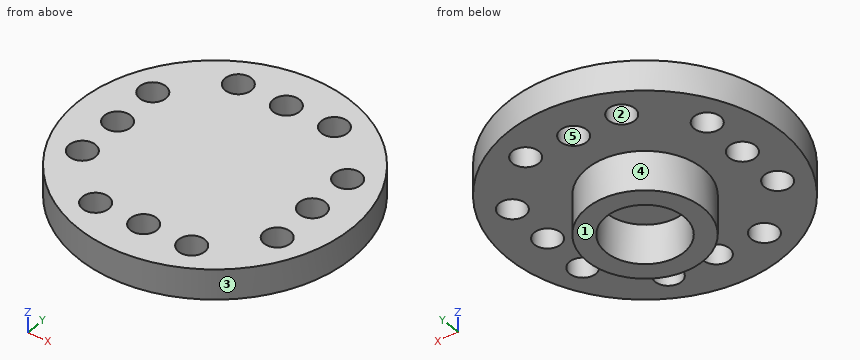
```python
from build123d import *

# Parameters (mm, degrees)
EXTRUDE_START       = 1
SKETCH_2_R          = 4.4
SKETCH_2_R_2        = 2.95
EXTRUDE_2_DEPTH     = 3
SKETCH_3_R          = 10.4
EXTRUDE_3_DEPTH     = 2.3
SKETCH_5_R          = 1
CUT_EXTRUDE_1_DEPTH = 2.3


with BuildPart() as part:
    # 스케치2 → 보스-돌출2 (new body)
    with BuildSketch(Plane.XY.offset(-4).offset(EXTRUDE_START)):
        with Locations((10.45, 0)):
            Circle(SKETCH_2_R)
        with Locations((10.45, 0)):
            Circle(SKETCH_2_R_2, mode=Mode.SUBTRACT)
    extrude(amount=EXTRUDE_2_DEPTH)

    # 스케치3 → 보스-돌출3 (add)
    with BuildSketch(Plane.XY):
        with Locations((10.45, 0)):
            Circle(SKETCH_3_R)
    extrude(amount=EXTRUDE_3_DEPTH)

    # 스케치5 → 컷-돌출1 (cut)
    with BuildSketch(Plane.XY.offset(2.3)):
        with Locations((10.45, 7.3)):
            Circle(SKETCH_5_R)
        with Locations((14.05, 7.3)):
            Circle(SKETCH_5_R)
        with Locations((6.85, 7.3)):
            Circle(SKETCH_5_R)
        with Locations((3.15, 0)):
            Circle(SKETCH_5_R)
        with Locations((3.15, 3.6)):
            Circle(SKETCH_5_R)
        with Locations((3.15, -3.6)):
            Circle(SKETCH_5_R)
        with Locations((10.45, -7.3)):
            Circle(SKETCH_5_R)
        with Locations((6.85, -7.3)):
            Circle(SKETCH_5_R)
        with Locations((14.05, -7.3)):
            Circle(SKETCH_5_R)
        with Locations((17.75, 0)):
            Circle(SKETCH_5_R)
        with Locations((17.75, -3.6)):
            Circle(SKETCH_5_R)
        with Locations((17.75, 3.6)):
            Circle(SKETCH_5_R)
    extrude(amount=-CUT_EXTRUDE_1_DEPTH, mode=Mode.SUBTRACT)


solid = part.part
```
Work out the finished part from the listing and answer in its coordinate system (mm). Face numbers are marked on the shaded views. A direction names the side the tool comes from. Round coordinates to 2 decimals unless told otherwise and drop trailing zeros. Loops run counter-clockwise (first coordinate to the right, second up) from the corner with the lowest first, then second, coordinate; pieces in that order, holes last.
(1) The mould has two halves that part along X. Classify the marked faces 1, 2 and 3: pulls with the +X half, pulls with the -X half, needs draft (parallel to the pull), parting line crosses it, or undercut.
Computed values:
face 1: needs draft
face 2: undercut
face 3: parting line crosses it
(2) The part is cut by section B-B, the plane x = 6.5. Give the vertices of the cut face in (y, z).
Computed values:
outline: (-9.62, 0) - (-8.24, 0) - (-8.24, 2.3) - (-9.62, 2.3) - close; (-6.36, 0) - (-1.94, 0) - (-1.94, -3) - (1.94, -3) - (1.94, 0) - (6.36, 0) - (6.36, 2.3) - (-6.36, 2.3) - close; (8.24, 0) - (9.62, 0) - (9.62, 2.3) - (8.24, 2.3) - close
(3) The part is cut by section D-D, the plane z = -2.4. Give the vertices of the cut face in (x, y), and give its area (3 significant figures).
Computed values:
outline: circle Ø8.8 at (10.45, 0); hole circle Ø5.9 at (10.45, 0)
area: 33.5 mm2
(4) Find the intervals of material crossed by L1, parallel to Y at x = 10.25, z = 1.6; L2, parallel to Y at x = 10.45, z = -2.05; L3, parallel to Y at x = 3.15, z = 1.2, in increasing order.
Computed values:
L1: y = -10.4 to -8.28, -6.32 to 6.32, 8.28 to 10.4
L2: y = -4.4 to -2.95, 2.95 to 4.4
L3: y = -7.41 to -4.6, -2.6 to -1, 1 to 2.6, 4.6 to 7.41
(5) The part is cut by section A-A, the plane y = 0. Give the vertices of the cut face in (x, z), and give its area (3 significant figures).
Computed values:
outline: (0.05, 0) - (2.15, 0) - (2.15, 2.3) - (0.05, 2.3) - close; (4.15, 0) - (6.05, 0) - (6.05, -3) - (7.5, -3) - (7.5, 0) - (13.4, 0) - (13.4, -3) - (14.85, -3) - (14.85, 0) - (16.75, 0) - (16.75, 2.3) - (4.15, 2.3) - close; (18.75, 0) - (20.85, 0) - (20.85, 2.3) - (18.75, 2.3) - close
area: 47.3 mm2
(6) For the marked faces 4 and 5, determine the directions among +Z, -Z, +X, -X, +Y, -Y from which every point of the face is accessible in a straight line to the end or side of a thin tool.
Computed values:
face 4: -Z
face 5: +Z, -Z
(7) The part is cut by section C-C, the plane x = 17.75. Give the vertices of the cut face in (y, z).
Computed values:
outline: (-7.41, 0) - (-4.6, 0) - (-4.6, 2.3) - (-7.41, 2.3) - close; (-2.6, 0) - (-1, 0) - (-1, 2.3) - (-2.6, 2.3) - close; (1, 0) - (2.6, 0) - (2.6, 2.3) - (1, 2.3) - close; (4.6, 0) - (7.41, 0) - (7.41, 2.3) - (4.6, 2.3) - close
(8) This flat-tipped pin is pushed along its axis until it touches: P1, Ø2.5, axis at x = 17.75, y = 0, coming from the -Z side. Where does it stop, or does it pass through?
Computed values:
P1: stops at z = 0
